Geometry check sheet. Reference: drawing and pictorial views, mm from the part's lowest x, y, z. A direction names the side the tool comes from. Give positions to 0.01 mm unless a question says otherwise; leave off trailing zeros. Order: outer loops, then holes, each group sorted by start corner. A loop starts at its lowest first (then second) coordinate and runs counter-clockwise, first axis right, second up. Notation, with made-up numbers: M 14,14.5 L 25,14.5 A29 cw 25,48.5 Z; hole C -1,-6 d10. An arc over 180 degrees is marked long. Answer as CSV lines item,"result".
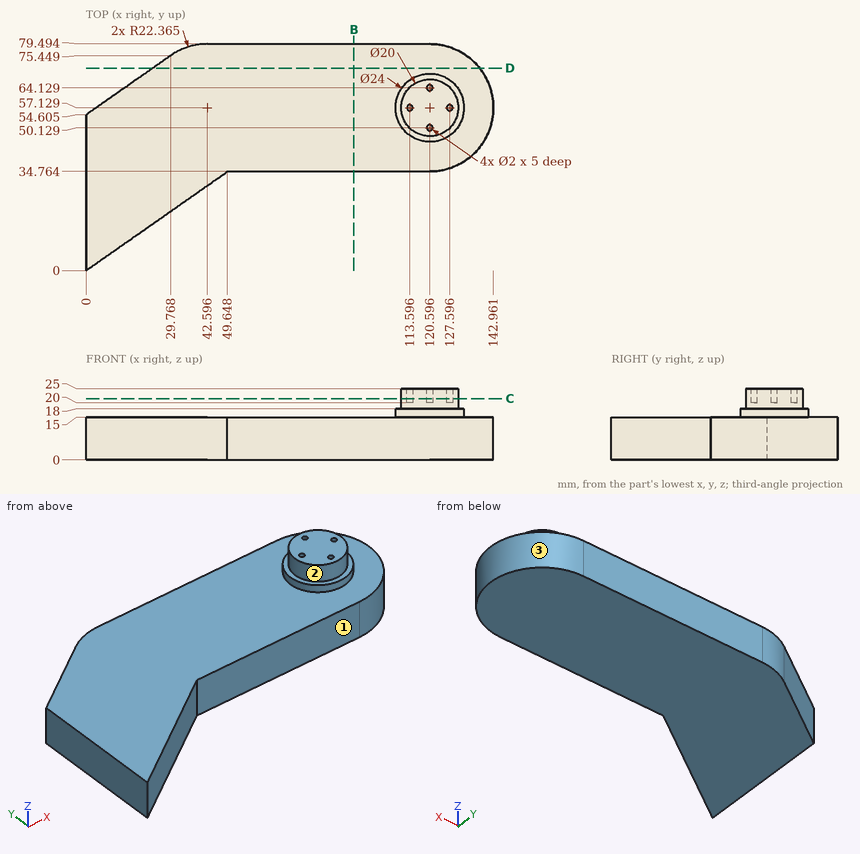
(1) Tool access check on the marked faces 1, 2 and 3. Record the directions out of +Z, -Z, +X, -X, +Y, -Y that give a thin tool (end or side, any length) a straight path to the whole face; none if there is none.
The answers:
face 1,"+Z, -Z, +X, -Y"
face 2,"+Z"
face 3,"+Z, -Z, +X"
(2) Material ranges on line 1 (Z direction, x = 33.5, y = 73); line 2 (Y direction, x = 107, z = 5); line 3 (X direction, y = 14, z = 6) (1 decimal), recorded low to high.
The answers:
line 1,"z = 0 to 15"
line 2,"y = 34.76 to 79.49"
line 3,"x = 0 to 20"
(3) Section check D-D on y = 71. Enter the section's corners in (x, z) (1 decimal), then the cut area to 3 significant figures.
The answers:
outline,"M 23.4,0 L 138.1,0 L 138.1,15 L 23.4,15 Z"
area,"1,720 mm2"
(4) Section check C-C on z = 21.5. Enter the section's corners in (x, y).
The answers:
outline,"C 120.6,57.13 d20; hole C 113.6,57.13 d2; hole C 120.6,50.13 d2; hole C 120.6,64.13 d2; hole C 127.6,57.13 d2"
(5) Gauge pin test, flat ends, axial feed: P1, Ø2, axis at x = 120, y = 64, coming from the +Z side; P2, Ø5, axis at y = 64, z = 12.5, coming from the +X side; P3, Ø24, axis at x = 71, y = 36.5, coming from the +Z side; P4, Ø3, axis at y = 44.5, z = 7, coming from the +X side (1 decimal). Record the tip position at first contact, or that the pin passes through.
The answers:
P1,"stops at z = 25"
P2,"stops at x = 142.53"
P3,"stops at z = 15"
P4,"stops at x = 140"
(6) Section check B-B on x = 94. Enter the section's corners in (y, z).
The answers:
outline,"M 34.76,0 L 79.49,0 L 79.49,15 L 34.76,15 Z"
